Build history of the part. All positions in model axes, mm. Give positions to 0.01 mm unless a question says otherwise; leave off trailing zeros. Write each loop counter-clockwise with the first axis right and the second up, starting at its lowest first coordinate (ties: lowest second). Pieces come first, ordered by that corner, then holes. Notation, with made-up numbers: (22.25, -24) -> (48.25, -24) arc R15 ccw to (48.25, -6) -> close; hole circle Ø8 at (-29.75, 24). An arc over 180 degrees is marked (long way). Put each result on its own line as item: value.
from build123d import *

# Parameters (mm, degrees)
SKETCH1_W           = 20
SKETCH1_H           = 70
SKETCH1_R           = 2
BOSS_EXTRUDE1_DEPTH = 1.5
SKETCH2_W           = 50
SKETCH2_H           = 40
BOSS_EXTRUDE2_DEPTH = 1.5
SKETCH3_R           = 2
CUT_EXTRUDE1_DEPTH  = 10
CHAMFER1_SIZE       = 8
FILLET1_R           = 10


with BuildPart() as part:
    # Sketch1 → Boss-Extrude1 (new body)
    with BuildSketch(Plane.XY):
        with Locations((-15.5, 0)):
            Rectangle(SKETCH1_W, SKETCH1_H)
        with Locations((-9, -12)):
            Circle(SKETCH1_R, mode=Mode.SUBTRACT)
        with Locations((-9, 12)):
            Circle(SKETCH1_R, mode=Mode.SUBTRACT)
        with Locations((-15, -18)):
            Circle(SKETCH1_R, mode=Mode.SUBTRACT)
        with Locations((-15, 18)):
            Circle(SKETCH1_R, mode=Mode.SUBTRACT)
        with Locations((-20.5, -24.571324751)):
            Circle(SKETCH1_R, mode=Mode.SUBTRACT)
        with Locations((-20.5, 24.571324751)):
            Circle(SKETCH1_R, mode=Mode.SUBTRACT)
    extrude(amount=BOSS_EXTRUDE1_DEPTH)

    # Sketch2 → Boss-Extrude2 (add)
    with BuildSketch(Plane.XY.offset(1.5)):
        with Locations((-0.5, -55)):
            Rectangle(SKETCH2_W, SKETCH2_H)
    boss_extrude2 = extrude(amount=-BOSS_EXTRUDE2_DEPTH)

    # Sketch3 → Cut-Extrude1 (cut)
    with BuildSketch(Plane.XY.offset(1.5)):
        with Locations((14.5, -69)):
            Circle(SKETCH3_R)
        with Locations((4.5, -69)):
            Circle(SKETCH3_R)
        with Locations((-5.5, -69)):
            Circle(SKETCH3_R)
        with Locations((-15.5, -69)):
            Circle(SKETCH3_R)
        with Locations((4.5, -59)):
            Circle(SKETCH3_R)
        with Locations((14.5, -59)):
            Circle(SKETCH3_R)
        with Locations((-15.5, -59)):
            Circle(SKETCH3_R)
        with Locations((-15.5, -49)):
            Circle(SKETCH3_R)
        with Locations((-15.5, -39)):
            Circle(SKETCH3_R)
    cut_extrude1 = extrude(amount=-CUT_EXTRUDE1_DEPTH, mode=Mode.SUBTRACT)

    # Mirror1: Boss-Extrude2, Cut-Extrude1 across plane
    add(boss_extrude2.mirror(Plane.ZX))
    add(cut_extrude1.mirror(Plane.ZX), mode=Mode.SUBTRACT)

    # Chamfer1
    chamfer1_edges = [part.edges().sort_by_distance(p)[0] for p in [
        (24.5, -75, 0.75),
        (24.5, -35, 0.75),
        (-25.5, -75, 0.75),
        (24.5, 35, 0.75),
        (-25.5, 75, 0.75),
        (24.5, 75, 0.75),
    ]]
    chamfer(chamfer1_edges, length=CHAMFER1_SIZE)

    # Fillet1
    fillet1_edges = [part.edges().sort_by_distance(p)[0] for p in [
        (-5.5, 35, 0.75),
        (-5.5, -35, 0.75),
    ]]
    fillet(fillet1_edges, radius=FILLET1_R)


solid = part.part
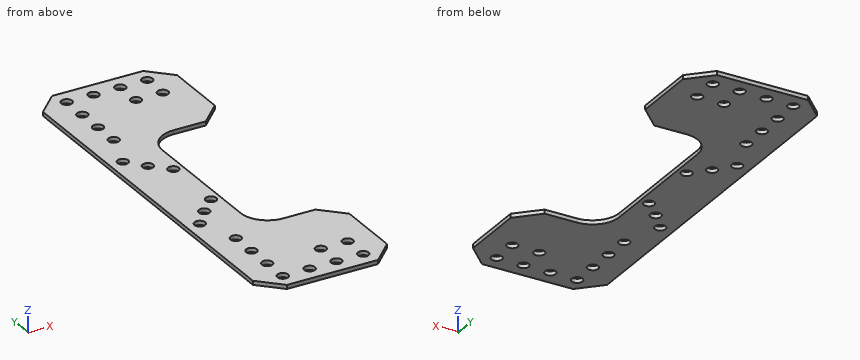
1) Slice it at A-A (x = 14.5). Write the cut outline in (y, z).
Filled sheet:
outline: (-75, 0) -> (-71, 0) -> (-71, 1.5) -> (-75, 1.5) -> close; (-67, 0) -> (-61, 0) -> (-61, 1.5) -> (-67, 1.5) -> close; (-57, 0) -> (-35, 0) -> (-35, 1.5) -> (-57, 1.5) -> close; (35, 0) -> (57, 0) -> (57, 1.5) -> (35, 1.5) -> close; (61, 0) -> (67, 0) -> (67, 1.5) -> (61, 1.5) -> close; (71, 0) -> (75, 0) -> (75, 1.5) -> (71, 1.5) -> close
2) Wall check: L1, parallel to Y at x = 14.5, z = 1; L2, parallel to Y at x = -9, z = 0.1; L3, parallel to Y at x = -8.5, z = 0.55. Give the ranges that are in metal, low to high.
Filled sheet:
L1: -75 to -71, -67 to -61, -57 to -35, 35 to 57, 61 to 67, 71 to 75
L2: -75 to -14, -10 to 10, 14 to 75
L3: -75 to -13.94, -10.06 to 10.06, 13.94 to 75
3) Slice it at D-D (x = -20.5). Write the cut outline in (y, z), plus the area to 3 significant figures.
Filled sheet:
outline: (-72, 0) -> (-26.57, 0) -> (-26.57, 1.5) -> (-72, 1.5) -> close; (-22.57, 0) -> (22.57, 0) -> (22.57, 1.5) -> (-22.57, 1.5) -> close; (26.57, 0) -> (72, 0) -> (72, 1.5) -> (26.57, 1.5) -> close
area: 204 mm2
4) Pin check, flat tip, straight feed: pin 1 (0.8 mm diameter, centred on y = -2, z = 0.5, fed in from +X). Stop position of the tip, or through.
Filled sheet:
pin 1: x = -5.5
5) Slice it at C-C (x = 21). Write the cut outline in (y, z), plus the area to 3 significant figures.
Filled sheet:
outline: (-70.5, 0) -> (-39.5, 0) -> (-39.5, 1.5) -> (-70.5, 1.5) -> close; (39.5, 0) -> (70.5, 0) -> (70.5, 1.5) -> (39.5, 1.5) -> close
area: 93.0 mm2
6) Slice it at B-B (y = -18). Write the cut outline in (x, z), plus the area to 3 significant figures.
Filled sheet:
outline: (-25.5, 0) -> (-17, 0) -> (-17, 1.5) -> (-25.5, 1.5) -> close; (-13, 0) -> (-5.5, 0) -> (-5.5, 1.5) -> (-13, 1.5) -> close
area: 24.0 mm2
